Design review of the part built by this model. Coordinates are the model's own, in mm. Give positions to 0.01 mm unless a question says otherwise; leave off trailing zeros. Write each loop counter-clockwise with the first axis right and the second up, starting at its lowest first coordinate (ties: lowest second). Pieces come first, ordered by that corner, then holes. Notation, with made-up numbers: (4.5, 8) -> (63.5, 8) arc R16 ccw to (63.5, 26) -> close; hole circle Ø4 at (86.5, 48). An arc over 180 degrees is marked (long way). Put each result on its own line as item: value. Start each with the question number.
Autodesk Inventor part; units mm, degrees
ref_plane "YZ Plane" through (0, 0, 0) normal (1, 0, 0) x (0, 1, 0)
ref_plane "XZ Plane" through (0, 0, 0) normal (0, 1, 0) x (-1, 0, 0)
ref_plane "XY Plane" through (0, 0, 0) normal (0, 0, 1) x (1, 0, 0)
sketch "Sketch1" plane through (0, 0, 0) normal (0, 1, 0) x (-1, 0, 0)
  circle A0 centre (0, 0) radius 2.413
  circle A1 centre (0, 50.8) radius 2.413
  line L0 (0, 50.8) -> (0, 0) construction
  circle A2 centre (11.3919, 12.7) radius 2.413
  circle A3 centre (11.3919, 0) radius 2.413
  circle A4 centre (-11.3919, 0) radius 2.413
  circle A5 centre (-11.3919, 12.7) radius 2.413
  line L1 (-11.3919, 0) -> (-11.3919, 12.7) construction
  line L2 (-11.3919, 12.7) -> (11.3919, 12.7) construction
  line L3 (1.5875, 55.2652) -> (15.5575, 47.1996)
  line L4 (-15.5575, 47.1996) -> (-1.5875, 55.2652)
  arc A6 (1.5875, 55.2652) -> (-1.5875, 55.2652) centre (0, 52.5156) ccw
  arc A7 (-15.5575, 47.1996) -> (-17.145, 44.45) centre (-13.97, 44.45) ccw
  arc A8 (17.145, 44.45) -> (15.5575, 47.1996) centre (13.97, 44.45) ccw
  line L5 (-17.145, 6.35) -> (-17.145, 44.45)
  line L6 (17.145, -4.7625) -> (17.145, 44.45)
  line L7 (17.145, -4.7625) -> (-17.145, -4.7625)
  line L8 (-17.145, 6.35) -> (-17.145, -4.7625)
  line L9 (13.97, 44.45) -> (-13.97, 44.45) construction
  point P0 (0, 25.4)
  point P1 (0, 56.1818)
  point P2 (26.6578, 40.7909)
  point P3 (26.6578, 10.0091)
  point P4 (-26.6578, 10.0091)
  point P5 (-26.6578, 40.7909)
  dimension "d1" = 4.826
  dimension "d2" = 50.8
  dimension "d3" = 4.826
  dimension "d4" = 4.826
  dimension "d5" = 12.7
  dimension "d6" = 11.3919
  dimension "d7" = 11.3919
  dimension "d8" = 0
  dimension "d9" = 4.826
  dimension "d10" = 4.826
  dimension "d11" = 11.3919
  dimension "d12" = 12.7
  dimension "d14" = 3.175
  dimension "d17" = 38.1
  dimension "d18" = 34.29
  dimension "d19" = 4.7625
  dimension "d20" = 6.35
  dimension "d21" = 49.2125
  dimension "d22" = 8.0656
extrude "Extrusion1" add sketch "Sketch1" along normal blind 3.175
fillet "Fillet1" radius 3.175 2 edges at (-17.145, 1.5875, -4.7625) (17.145, 1.5875, -4.7625)
equation "\"d7\" = d6"
equation "\"d11\" = d6"
equation "\"d21\" = d20 + d19 + d17"
properties part number "Roller Pneumatic Back Connector (Custom)" material "Aluminum 6061"
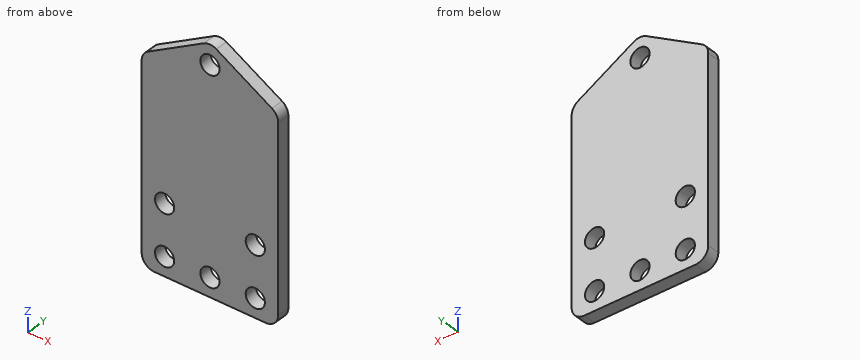
Q1. Take a section at A-A on z = 0. Give the boundary of the cut face in (x, y) (3 decimals), then the cut area to 3 significant figures.
Q2. Take a section at B-B on x = 0. Give the boundary of the cut face in (y, z) (1 decimal), then the cut area to 3 significant figures.
Q3. To check wall thickness, follow probe 1 along Z at (x, y) = (0, 0.95); probe 2 along Z at (x, y) = (-12.5, 0.75); probe 3 along X at (y, z) = (2.8, 51.5). State the ranges of each line that lie inside material, in increasing order. Write a range as from..to.
Q4. For pin 1 (4 mm diameter, centred on x = 11.39, z = 0, fed in from +Y); pin 2 (6.5 mm diameter, centred on x = -11.39, z = 12.7, fed in from +Y) (3 decimals), all flat-tipped, find the tip position at first contact; note any pin that passes through.
Q5. Take a section at C-C on z = 12.7. Give the boundary of the cut face in (x, y) (3 decimals), then the cut area to 3 significant figures.
Q6. Take a section at D-D on y = 1.2. State how many separate pieces and enclosed holes the cut face has, then the cut area to 3 significant figures.
Result:
1. outline: (-17.145, 0) -> (-13.805, 0) -> (-13.805, 3.175) -> (-17.145, 3.175) -> close; (-8.979, 0) -> (-2.413, 0) -> (-2.413, 3.175) -> (-8.979, 3.175) -> close; (2.413, 0) -> (8.979, 0) -> (8.979, 3.175) -> (2.413, 3.175) -> close; (13.805, 0) -> (17.145, 0) -> (17.145, 3.175) -> (13.805, 3.175) -> close
1. area: 62.9 mm^2
2. outline: (0, -4.8) -> (3.2, -4.8) -> (3.2, -2.4) -> (0, -2.4) -> close; (0, 2.4) -> (3.2, 2.4) -> (3.2, 48.4) -> (0, 48.4) -> close; (0, 53.2) -> (3.2, 53.2) -> (3.2, 55.7) -> (0, 55.7) -> close
2. area: 161 mm^2
3. probe 1: z = -4.76..-2.41, 2.41..48.39, 53.21..55.69
3. probe 2: z = -4.76..-2.14, 2.14..10.56, 14.84..48.96
3. probe 3: x = -8.11..-2.31, 2.31..8.11
4. pin 1: passes through
4. pin 2: stops at y = 3.175
5. outline: (-17.145, 0) -> (-13.805, 0) -> (-13.805, 3.175) -> (-17.145, 3.175) -> close; (-8.979, 0) -> (8.979, 0) -> (8.979, 3.175) -> (-8.979, 3.175) -> close; (13.805, 0) -> (17.145, 0) -> (17.145, 3.175) -> (13.805, 3.175) -> close
5. area: 78.2 mm^2
6. separate pieces: 1
6. enclosed holes: 6
6. area: 1,800 mm^2
